Here's how the part is built. I have some questions about the finished solid (model axes, mm). A direction names the side the tool comes from. Round coordinates to 2 decimals unless told otherwise and drop trailing zeros. Write each loop counter-clockwise with the first axis right and the second up, starting at its lowest first coordinate (ties: lowest second). Pieces come first, ordered by that corner, then holes. Notation, with made-up numbers: (86, 2.5) -> (126, 2.5) arc R23 ccw to (126, 33.5) -> close; hole circle Ø6 at (-37.75, -7.5). An arc over 180 degrees is marked (long way). Answer as CSV lines item,"result".
from build123d import *

# Parameters (mm, degrees)
SCHIZZO2_R               = 4.5
TAGLIO_ESTRUSIONE1_DEPTH = 94.653617122
SCHIZZO3_W               = 75.498344352
SCHIZZO3_H               = 30
TAGLIO_ESTRUSIONE2_DEPTH = 95.207218407


with BuildPart() as part:
    # Schizzo1 → Rivoluzione1 (revolve)
    with BuildSketch(Plane.XY, mode=Mode.PRIVATE) as rivoluzione1_sk:
        Polygon((0, 0), (0, 5), (6, 5), (6, 35), (11, 35), (11, 16), (14.5, 16), (14.5, 13.75), (18, 13.75), (18, 16), (21, 16), (21, 11), (12, 11), (12, -2), (10, -2), (10, 0), align=None)
    revolve(rivoluzione1_sk.sketch.rotate(Axis((-8.306759574, -20, 0), (1, 0, 0)), 90), axis=Axis((-8.306759574, -20, 0), (1, 0, 0)))

    # Schizzo2 → Taglio-Estrusione1 (cut, through all)
    with BuildSketch(Plane(origin=(11, 0, 0), x_dir=(0, 0, -1), z_dir=(1, 0, 0))):
        with Locations((0, 25)):
            Circle(SCHIZZO2_R)
        with Locations((88.334591186, -128)):
            Circle(SCHIZZO2_R)
        with Locations((-88.334591186, -128)):
            Circle(SCHIZZO2_R)
        with Locations((38.97114317, -42.5)):
            Circle(SCHIZZO2_R)
        with Locations((-38.97114317, -42.5)):
            Circle(SCHIZZO2_R)
    extrude(amount=-TAGLIO_ESTRUSIONE1_DEPTH, mode=Mode.SUBTRACT)

    # Schizzo3 → Taglio-Estrusione2 (cut, through all)
    with BuildSketch(Plane.ZY.offset(-6)):
        with Locations((0, -75)):
            Rectangle(SCHIZZO3_W, SCHIZZO3_H)
    extrude(amount=-TAGLIO_ESTRUSIONE2_DEPTH, mode=Mode.SUBTRACT)


solid = part.part
Item 1: Suppose I cut it at B-B, the plane z = -39.5. List the corners of the cut face in (x, y) for me, then the cut area to 3 significant figures.
Results found:
outline,"(6, -58.27) -> (11, -58.27) -> (11, -46.97) -> (6, -46.97) -> close; (6, -38.03) -> (11, -38.03) -> (11, 18.27) -> (6, 18.27) -> close"
area,"338 mm²"
Item 2: I need wall thicknesses on L1, parallel to X at y = -15.5, z = -35.5; L2, parallel to X at y = -16.5, z = -22; L3, parallel to X at y = -13.5, z = 32.5. Which ranges of each line are inside material? Lowest first, please.
Results found:
L1,"x = 6 to 14.5, 18 to 21"
L2,"x = 0 to 12"
L3,"x = 6 to 21"
Item 3: Will these pins go through, and if not, where does the flat tip stop? pin 1 (2 mm diameter, centred on x = 8.5, y = -35.5, fed in from +Z); pin 2 (14.5 mm diameter, centred on y = -42.5, z = -38.97, fed in from +X); pin 3 (12 mm diameter, centred on y = -31, z = -21.5, fed in from +X).
Results found:
pin 1,"stops at z = 53.05"
pin 2,"stops at x = 11"
pin 3,"stops at x = 12"
Item 4: For faces 4 (the flat face through (12, -7, 13)), 5 (the flat face through (14.5, -52.2, -10.8)), 6 (the cylindrical face through (4.93, -0.476, -4.336)), which set-ups out of +Z, -Z, +X, -X, +Y, -Y let a thin tool reach every point of the face, with its end or its side?
Results found:
face 4,"+X"
face 5,"none"
face 6,"-X"
Item 5: Suppose I cut it at D-D, the plane y = -42.5. State how many separate pieces and enclosed holes the cut face has, then the cut area to 3 significant figures.
Results found:
separate pieces,"3"
enclosed holes,"0"
area,"700 mm²"
Item 6: Suppose I cut it at C-C, the plane x = 8. List the corners of the cut face in (y, z) for me.
Results found:
outline,"(-60, -37.75) arc R55 ccw (long way) to (-60, 37.75) -> close; hole circle Ø9 at (-42.5, -38.97); hole circle Ø9 at (-42.5, 38.97); hole circle Ø40 at (-20, 0); hole circle Ø9 at (25, 0)"
Item 7: If we mould it in two halves opening along Z, with no side actions, what happens to faces 1 (the flat face through (6, 8, 1)), 2 (the cylindrical face through (8.54, -46.49, 36.89)), 3 (the cylindrical face through (16.274, 12.947, -7.316))? For each: pulls with the +Z half, pulls with the -Z half, needs draft (parallel to the pull), parting line crosses it, or undercut.
Results found:
face 1,"needs draft"
face 2,"undercut"
face 3,"parting line crosses it"
